The model under review builds one solid part; all positions refer to its coordinate system, in mm. Face numbers are marked on the shaded views. A direction names the side the tool comes from. Coordinates: 2 decimals unless noted, no trailing zeros. Loops run counter-clockwise (first coordinate to the right, second up) from the corner with the lowest first, then second, coordinate; pieces in that order, holes last. Notation, with made-up numbers: M 76,-11 L 93,-11 A19 cw 93,22 Z; hole C 27,-25 d8. An arc over 180 degrees is marked long. Return JSON: item names as keys, results as strings.
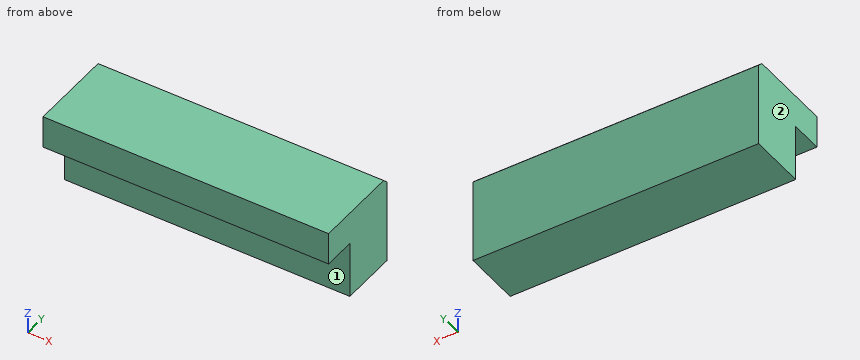
```python
from build123d import *

# Parameters (mm, degrees)
F0_W     = 70.0024
F0_H     = 8.001
F1_DEPTH = 21.9964
F0_H_2   = 13.9954
F2_DEPTH = 13.9954
F3_SIZE  = 1.27


with BuildPart() as f1:
    # F0 (on Front) → F1 (new body)
    with BuildSketch(Plane.XZ):
        with Locations((0, 6.9977)):
            Rectangle(F0_W, F0_H)
    extrude(amount=F1_DEPTH)

    # F0 (on Front) → F2 (join)
    with BuildSketch(Plane.XZ):
        with Locations((0, -4.0005)):
            Rectangle(F0_W, F0_H_2)
    extrude(amount=F2_DEPTH)

    # F3
    f3_edges = [f1.edges().sort_by_distance(p)[0] for p in [
        (0, 0, 10.9982),
    ]]
    chamfer(f3_edges, length=F3_SIZE)


solid = f1.part
```
1. Machinability: for the marked faces 1 and 2, which of the approach directions +Z, -Z, +X, -X, +Y, -Y give a long, thin tool a straight path to every point of the face, cutting with its end or side? Answer none if there is none.
Check values:
{"face 1": "-Z, +X, -X, -Y", "face 2": "+Z, -Z, -X, +Y, -Y"}
2. Add section B-B on y = -15.5. Give the boundary of the cut face in (x, z).
Check values:
{"outline": "M -35,3 L 35,3 L 35,11 L -35,11 Z"}
3. To check wall thickness, follow line 1 (Y direction, x = 13, z = -2.5); line 2 (Z direction, x = 3.5, y = -17); line 3 (Z direction, x = 22.5, y = -0.75). State the ranges of each line that lie inside material, in increasing order.
Check values:
{"line 1": "-14 to 0", "line 2": "3 to 11", "line 3": "-11 to 10.48"}
4. Add section C-C on z = -7.5. Give the boundary of the cut face in (x, y).
Check values:
{"outline": "M -35,-14 L 35,-14 L 35,0 L -35,0 Z"}
5. Add section A-A on x = 0. Give the boundary of the cut face in (y, z).
Check values:
{"outline": "M -22,3 L -14,3 L -14,-11 L 0,-11 L 0,9.73 L -1.27,11 L -22,11 Z"}
6. Insertion check: pin 1 Ø6.5 at (x, y) = (6, -17.5) entering from -Z. The pin has a flat end and moves straight along its axis. Give the tip position at first contact, or say it passes through.
Check values:
{"pin 1": "z = 3"}
